For this review, take the finished solid that the model builds, in its own axes (mm). A direction names the side the tool comes from. Give positions to 0.01 mm unless a question says otherwise; leave off trailing zeros. Write each loop counter-clockwise with the first axis right and the second up, starting at its lowest first coordinate (ties: lowest second). Pieces come first, ordered by that corner, then holes. Notation, with made-up numbers: (-12.5, -26) -> (6.5, -26) arc R14 cw to (6.5, -9) -> close; hole circle Ø10 at (69, -13.5). An arc over 180 degrees is marked (long way). Write item = value, one per line.
```python
from build123d import *

# Parameters (mm, degrees)
SKETCH1_W           = 70
SKETCH1_H           = 70
BOSS_EXTRUDE1_DEPTH = 5
SKETCH2_R           = 25.5
SKETCH2_R_2         = 2
CUT_EXTRUDE3_DEPTH  = 2
SKETCH3_R           = 2
CUT_EXTRUDE4_DEPTH  = 10
SKETCH4_R           = 2
CUT_EXTRUDE5_DEPTH  = 10
SKETCH5_R           = 0.5
CUT_EXTRUDE7_DEPTH  = 10


with BuildPart() as part:
    # Sketch1 → Boss-Extrude1 (new body)
    with BuildSketch(Plane(origin=(0, 0, 0), x_dir=(1, 0, 0), z_dir=(0, 1, 0))):
        Rectangle(SKETCH1_W, SKETCH1_H)
    extrude(amount=BOSS_EXTRUDE1_DEPTH)

    # Sketch2 → Cut-Extrude3 (cut)
    with BuildSketch(Plane.XZ):
        with Locations(Location((0, 0, 0), (0, 0, 270))):
            Circle(SKETCH2_R)
        with Locations(Location((-18.5, 0, 0), (0, 0, 270))):
            Circle(SKETCH2_R_2, mode=Mode.SUBTRACT)
        with Locations(Location((18.5, 0, 0), (0, 0, 90))):
            Circle(SKETCH2_R_2, mode=Mode.SUBTRACT)
    extrude(amount=-CUT_EXTRUDE3_DEPTH, mode=Mode.SUBTRACT)

    # Sketch3 → Cut-Extrude4 (cut)
    with BuildSketch(Plane.XZ):
        with Locations(Location((18.5, 0, 0), (0, 0, 270))):
            Circle(SKETCH3_R)
    extrude(amount=-CUT_EXTRUDE4_DEPTH, mode=Mode.SUBTRACT)

    # Sketch4 → Cut-Extrude5 (cut)
    with BuildSketch(Plane(origin=(0, 0, 0), x_dir=(-1, 0, 0), z_dir=(0, -1, 0))):
        with Locations(Location((18.5, 0, 0), (0, 0, 90))):
            Circle(SKETCH4_R)
    extrude(amount=-CUT_EXTRUDE5_DEPTH, mode=Mode.SUBTRACT)

    # Sketch5 → Cut-Extrude7 (cut)
    with BuildSketch(Plane(origin=(0, 2, 0), x_dir=(-1, 0, 0), z_dir=(0, -1, 0))):
        with Locations(Location((4, 0, 0), (0, 0, 90))):
            Circle(SKETCH5_R)
    extrude(amount=-CUT_EXTRUDE7_DEPTH, mode=Mode.SUBTRACT)


solid = part.part
```
(1) Take a section at A-A (x = 0). Write out the cut boundary in (y, z).
Answers below:
outline = (0, -35) -> (5, -35) -> (5, 35) -> (0, 35) -> (0, 25.5) -> (2, 25.5) -> (2, -25.5) -> (0, -25.5) -> close
(2) Take a section at B-B (y = 0.8). Write out the cut boundary in (x, z), plus the area to 3 significant figures.
Answers below:
outline = (-35, -35) -> (35, -35) -> (35, 35) -> (-35, 35) -> close; hole circle Ø51 at (0, 0)
area = 2,860 mm^2
(3) For pin 1 (6 mm diameter, centred on x = 18.5, z = 0.5, fed in from -Y), flat-tipped, find the tip position at first contact; note if it passes through.
Answers below:
pin_1 = 2
(4) Tool access review of faces 1 (the face through (-24.9, 1, 5.5)), 2 (the face through (0, 2, 35)): name each direction out of +Z, -Z, +X, -X, +Y, -Y from which nothing blocks a thin tool from reaching the whole face with its end or side.
Answers below:
face_1 = -Y
face_2 = +Z, +X, -X, +Y, -Y
(5) Take a section at C-C (z = 14). Write out the cut boundary in (x, y).
Answers below:
outline = (-35, 0) -> (-21.31, 0) -> (-21.31, 2) -> (21.31, 2) -> (21.31, 0) -> (35, 0) -> (35, 5) -> (-35, 5) -> close
(6) To check wall thickness, follow probe 1 along X at (y, z) = (3.35, 0); probe 2 along X at (y, z) = (1.65, 0); probe 3 along Y at (x, z) = (-3.5, -8.5). State the ranges of each line that lie inside material, in increasing order.
Answers below:
probe_1 = -35 to -20.5, -16.5 to -4.5, -3.5 to 16.5, 20.5 to 35
probe_2 = -35 to -25.5, 25.5 to 35
probe_3 = 2 to 5
(7) Take a section at D-D (x = 18.5). Write out the cut boundary in (y, z), plus the area to 3 significant figures.
Answers below:
outline = (0, -35) -> (5, -35) -> (5, -2) -> (2, -2) -> (2, -17.55) -> (0, -17.55) -> close; (0, 17.55) -> (2, 17.55) -> (2, 2) -> (5, 2) -> (5, 35) -> (0, 35) -> close
area = 268 mm^2
(8) The part is to be moulded in two halves that separate along Z. For faces 3 (the face through (0, 5, 0)), 4 (the face through (0, 2, -35)), 5 (the face through (0, 2, 0)), say which applies: released by +Z, released by -Z, zero draft, split by the parting line, or undercut.
Answers below:
face_3 = zero draft
face_4 = released by -Z
face_5 = undercut
